from build123d import *

# Parameters (mm, degrees)
Y_KSEKLIK_EKSTR_ZYON1_DEPTH      = 315
Y_KSEKLIK_EKSTR_ZYON1_DEPTH_BACK = 315
IZIM1_W                          = 26
IZIM1_H                          = 26
KES_EKSTR_ZYON1_DEPTH            = 250
KES_EKSTR_ZYON1_DEPTH_BACK       = 250


with BuildPart() as part:
    # Çizim1 → Yükseklik-Ekstrüzyon1 (new, two sides: drawn at the far end of the back side and taken through both)
    with BuildSketch(Plane.XY.offset(-Y_KSEKLIK_EKSTR_ZYON1_DEPTH_BACK)):
        with BuildLine():
            Line((-13, 15), (13, 15))
            ThreePointArc((13, 15), (14.414213562, 14.414213562), (15, 13))
            Line((15, 13), (15, -13))
            ThreePointArc((15, -13), (14.414213562, -14.414213562), (13, -15))
            Line((13, -15), (-13, -15))
            ThreePointArc((-13, -15), (-14.414213562, -14.414213562), (-15, -13))
            Line((-15, -13), (-15, 13))
            ThreePointArc((-15, 13), (-14.414213562, 14.414213562), (-13, 15))
        make_face()
        Rectangle(IZIM1_W, IZIM1_H, mode=Mode.SUBTRACT)
    extrude(amount=Y_KSEKLIK_EKSTR_ZYON1_DEPTH + Y_KSEKLIK_EKSTR_ZYON1_DEPTH_BACK)

    # Çizim2 → Kes-Ekstrüzyon1 (cut, two sides: drawn at the far end of the back side and taken through both)
    with BuildSketch(Plane(origin=(0, 0, 0), x_dir=(1, 0, 0), z_dir=(0, 1, 0)).offset(-KES_EKSTR_ZYON1_DEPTH_BACK)):
        Polygon((15, 315), (-15, 285), (-15, 315), align=None)
        Polygon((15, -315), (-15, -285), (-15, -315), align=None)
    extrude(amount=KES_EKSTR_ZYON1_DEPTH + KES_EKSTR_ZYON1_DEPTH_BACK, mode=Mode.SUBTRACT)


solid = part.part
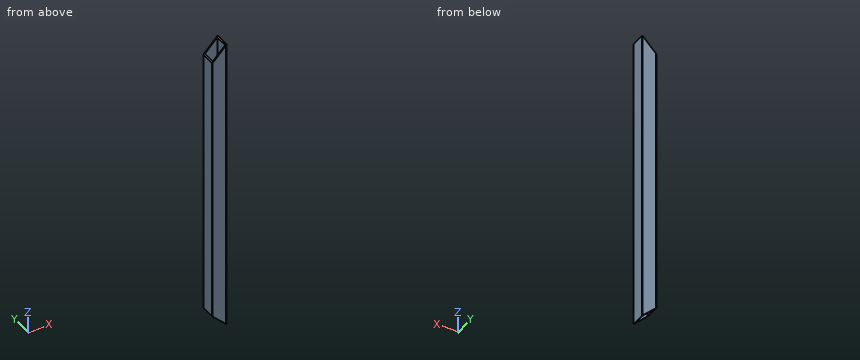
Model file for the job. Use its own axes, mm. Coordinates: 2 decimals unless noted, no trailing zeros. Order: outer loops, then holes, each group sorted by start corner. A loop starts at its lowest first (then second) coordinate and runs counter-clockwise, first axis right, second up. Notation, with made-up numbers: M -23.5,24 L 21.5,24 A16 cw 21.5,35 Z; hole C 49,15.5 d2. An arc over 180 degrees is marked long. Return JSON: item names as keys, results as strings.
1. Saw through at C-C (y = 1). Give the cut face in (x, z).
Ans:
{"outline": "M -15,-285 L -13,-287 L -13,287 L -15,285 Z; M 13,-313 L 15,-315 L 15,315 L 13,313 Z"}
2. Saw through at B-B (z = -5). Give the cut face in (x, y).
Ans:
{"outline": "M -15,-13 A2 ccw -13,-15 L 13,-15 A2 ccw 15,-13 L 15,13 A2 ccw 13,15 L -13,15 A2 ccw -15,13 Z; hole M -13,-13 L 13,-13 L 13,13 L -13,13 Z"}
3. Drill centre lines: probe 1 along Y at (x, z) = (11, -156); probe 2 along Y at (x, z) = (13.75, 168). Where is each one in solid material? Low to high.
Ans:
{"probe 1": "-15 to -13, 13 to 15", "probe 2": "-14.85 to 14.85"}
4. Flat gauge pins, fed straight in: pin 1 (10 mm diameter, centred on x = -7, y = 2, fed in from -Z); pin 2 (10 mm diameter, centred on x = -1.5, y = -11.5, fed in from +Z). Where does each tip first touch, or does it go through?
Ans:
{"pin 1": "through", "pin 2": "z = 303.27"}
5. Saw through at A-A (x = 1.75). Give the cut face in (y, z).
Ans:
{"outline": "M -15,-301.75 L -13,-301.75 L -13,301.75 L -15,301.75 Z; M 13,-301.75 L 15,-301.75 L 15,301.75 L 13,301.75 Z"}
